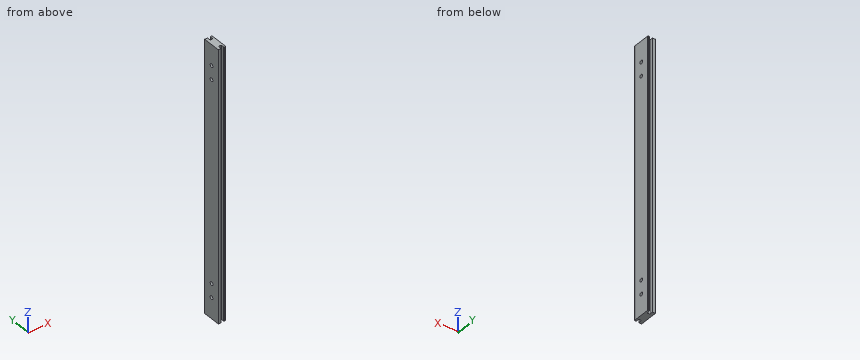
```python
from build123d import *

# Parameters (mm, degrees)
BOSS_EXTRUDE1_DEPTH = 195
CUT_EXTRUDE1_REACH  = 197.682
SKETCH4_R           = 2.5
FILLET1_R           = 1


with BuildPart() as part:
    # Sketch3 → Boss-Extrude1 (new, symmetric)
    with BuildSketch(Plane.XY):
        with BuildLine():
            Line((-6, 12.5), (-6, -12.5))
            Line((-6, -12.5), (-2, -12.5))
            Line((-2, -12.5), (-2, -8.5))
            ThreePointArc((-2, -8.5), (-1.707106781, -7.792893219), (-1, -7.5))
            Line((-1, -7.5), (1, -7.5))
            ThreePointArc((1, -7.5), (1.707106781, -7.792893219), (2, -8.5))
            Line((2, -8.5), (2, -12.5))
            Line((2, -12.5), (4.5, -12.5))
            Line((4.5, -12.5), (4.5, 12.5))
            Line((4.5, 12.5), (2, 12.5))
            Line((2, 12.5), (2, 8.5))
            ThreePointArc((2, 8.5), (1.707106781, 7.792893219), (1, 7.5))
            Line((1, 7.5), (-1, 7.5))
            ThreePointArc((-1, 7.5), (-1.707106781, 7.792893219), (-2, 8.5))
            Line((-2, 8.5), (-2, 12.5))
            Line((-2, 12.5), (-6, 12.5))
        make_face()
    extrude(amount=BOSS_EXTRUDE1_DEPTH, both=True)

    # Sketch4 → Cut-Extrude1 (cut, up to next)
    with BuildSketch(Plane.ZY.offset(6), mode=Mode.PRIVATE) as cut_extrude1_sk1:
        with Locations((-165, 0)):
            Circle(SKETCH4_R)
    cut_extrude1_tool1 = extrude(cut_extrude1_sk1.sketch, amount=-CUT_EXTRUDE1_REACH, mode=Mode.PRIVATE) & part.part
    # Sketch4 → Cut-Extrude1 (cut, up to next)
    with BuildSketch(Plane.ZY.offset(6), mode=Mode.PRIVATE) as cut_extrude1_sk2:
        with Locations((-145, 0)):
            Circle(SKETCH4_R)
    cut_extrude1_tool2 = extrude(cut_extrude1_sk2.sketch, amount=-CUT_EXTRUDE1_REACH, mode=Mode.PRIVATE) & part.part
    # Sketch4 → Cut-Extrude1 (cut, up to next)
    with BuildSketch(Plane.ZY.offset(6), mode=Mode.PRIVATE) as cut_extrude1_sk3:
        with Locations((165, 0)):
            Circle(SKETCH4_R)
    cut_extrude1_tool3 = extrude(cut_extrude1_sk3.sketch, amount=-CUT_EXTRUDE1_REACH, mode=Mode.PRIVATE) & part.part
    # Sketch4 → Cut-Extrude1 (cut, up to next)
    with BuildSketch(Plane.ZY.offset(6), mode=Mode.PRIVATE) as cut_extrude1_sk4:
        with Locations((145, 0)):
            Circle(SKETCH4_R)
    cut_extrude1_tool4 = extrude(cut_extrude1_sk4.sketch, amount=-CUT_EXTRUDE1_REACH, mode=Mode.PRIVATE) & part.part
    add(cut_extrude1_tool1.solids().sort_by_distance((-6, 0, -165))[0], mode=Mode.SUBTRACT)
    add(cut_extrude1_tool2.solids().sort_by_distance((-6, 0, -145))[0], mode=Mode.SUBTRACT)
    add(cut_extrude1_tool3.solids().sort_by_distance((-6, 0, 165))[0], mode=Mode.SUBTRACT)
    add(cut_extrude1_tool4.solids().sort_by_distance((-6, 0, 145))[0], mode=Mode.SUBTRACT)

    # Fillet1
    fillet1_edges = [part.edges().sort_by_distance(p)[0] for p in [
        (2, 12.5, 0),
        (4.5, 12.5, 0),
        (4.5, -12.5, 0),
        (2, -12.5, 0),
    ]]
    fillet(fillet1_edges, radius=FILLET1_R)


solid = part.part
```
CAD build for the part. Positions are in the model's coordinates, mm. Round coordinates to 2 decimals unless told otherwise and drop trailing zeros. Loops run counter-clockwise (first coordinate to the right, second up) from the corner with the lowest first, then second, coordinate; pieces in that order, holes last. Notation, with made-up numbers: M 37,25.5 L 95,25.5 A28 cw 95,49.5 Z; hole C 48,-17.5 d6. An arc over 180 degrees is marked long. Use a Markdown table: item, result. Add a question column.
(1) Flat gauge pins, fed straight in: pin 1 (3 mm diameter, centred on x = 0, z = 3, fed in from +Y); pin 2 (1.6 mm diameter, centred on x = -0.5, z = 21.5, fed in from -Y); pin 3 (1 mm diameter, centred on x = 0, z = -92, fed in from +Y). Where does each tip first touch, or does it go through?
(2) Cut at A-A (z = -25). Give the cut face in (x, y).
(3) Drill centre lines: line 1 (X direction, y = 9.25, z = 108); line 2 (Y direction, x = 0.25, z = -165); line 3 (Z direction, x = -1.5, y = 1.75). Where is each one in solid material? Low to high.
Geometry says:
| question | item | result |
|---|---|---|
| 1 | pin 1 | stops at y = 7.63 |
| 1 | pin 2 | stops at y = -7.55 |
| 1 | pin 3 | stops at y = 7.5 |
| 2 | outline | M -6,-12.5 L -2,-12.5 L -2,-8.5 A1 cw -1,-7.5 L 1,-7.5 A1 cw 2,-8.5 L 2,-11.5 A1 ccw 3,-12.5 L 3.5,-12.5 A1 ccw 4.5,-11.5 L 4.5,11.5 A1 ccw 3.5,12.5 L 3,12.5 A1 ccw 2,11.5 L 2,8.5 A1 cw 1,7.5 L -1,7.5 A1 cw -2,8.5 L -2,12.5 L -6,12.5 Z |
| 3 | line 1 | x = -6 to -2, 2 to 4.5 |
| 3 | line 2 | y = -7.5 to -2.5, 2.5 to 7.5 |
| 3 | line 3 | z = -195 to -166.79, -163.21 to -146.79, -143.21 to 143.21, 146.79 to 163.21, 166.79 to 195 |
